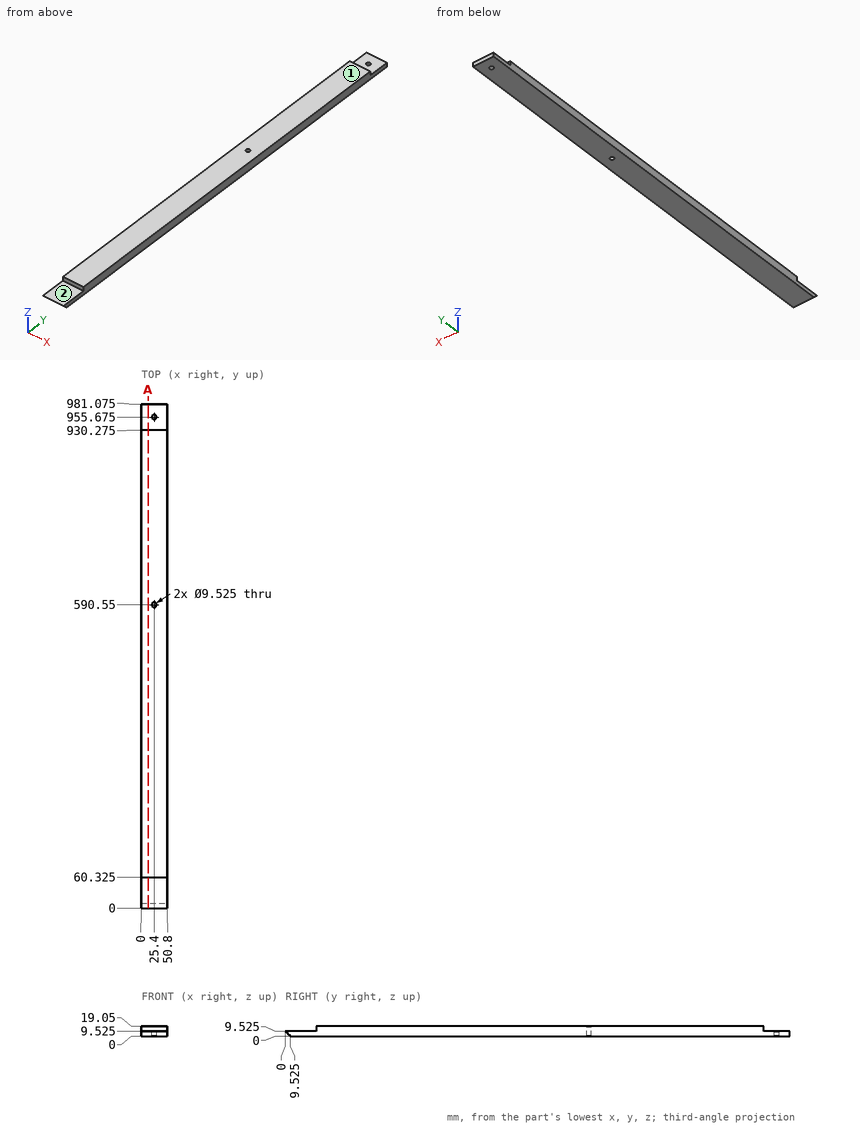
The figure shows three views and two pictorial views of one solid part (mm, origin at its lowest corner). Answer the questions. A direction names the side the tool comes from. Give positions to 0.01 mm unless a question says otherwise; leave off trailing zeros. Write each loop counter-clockwise with the first axis right and the second up, starting at its lowest first coordinate (ties: lowest second). Pieces come first, ordered by that corner, then holes. Notation, with made-up numbers: (71, -17.5) - (128, -17.5) arc R20 cw to (128, -1.5) - close; hole circle Ø10 at (-38.5, -6). An arc over 180 degrees is marked (long way). Return JSON: item names as keys, results as strings.
Q1. For the marked faces 1 and 2, determine the directions among +Z, -Z, +X, -X, +Y, -Y from which every point of the face is accessible in a straight line to the end or side of a thin tool.
Reply:
{"face 1": "+Z, +X, -X, +Y, -Y", "face 2": "+Z, +X, -X, -Y"}
Q2. Consider line 1 along Y through (x, z) = (25.4, 13.75) (1 decimal); line 2 along X through (y, z) = (590.55, 10.75); line 3 along Y through (x, z) = (25.4, 7.25) (1 decimal). Determine where each line is inside the solid, lowest interval first. Write a range as [from, to].
Reply:
{"line 1": "[60.3, 585.8], [595.3, 930.3]", "line 2": "[0, 20.64], [30.16, 50.8]", "line 3": "[2.3, 585.8], [595.3, 950.9], [960.4, 981.1]"}
Q3. Given P1, Ø7.5, axis at x = 36.5, z = 12, coming from the -Y side; P2, Ø7.5, axis at x = 17.5, z = 15, coming from the +Y side (3 decimals); P3, Ø15, axis at x = 15.5, y = 945, coming from the +Z side (3 decimals), each flat-ended and moving along its own axis, determine where each tip first touches the part or whether it passes through.
Reply:
{"P1": "y = 0", "P2": "y = 930.275", "P3": "z = 9.525"}
Q4. A cutting plane is placed at A-A, the plane x = 13. Determine the outline of the cut face in (y, z) (3 decimals), and give its area (3 significant figures).
Reply:
{"outline": "(0, 9.525) - (9.525, 0) - (981.075, 0) - (981.075, 9.525) - (930.275, 9.525) - (930.275, 19.05) - (60.325, 19.05) - (60.325, 9.525) - close", "area": "17,600 mm²"}
